Work out the finished part from the listing and answer in its coordinate system (mm). Round coordinates to 2 decimals unless told otherwise and drop trailing zeros. Loops run counter-clockwise (first coordinate to the right, second up) from the corner with the lowest first, then second, coordinate; pieces in that order, holes last. Notation, with made-up numbers: (23.5, -24) -> (72.5, -24) arc R23 ccw to (72.5, -1) -> close; hole circle Ø10 at (4.25, 24). An arc over 180 degrees is marked (long way). Use CSV: the item, a comma, the result in double quotes. Start each with the question number.
Autodesk Fusion 360 part; units mm, degrees
sketch "Esquisse1" plane through (0, 0, 0) normal (0, 0, 1) x (1, 0, 0)
  line L0 (-15, 10) -> (15, 10)
  line L1 (15, 10) -> (15, 0)
  line L2 (15, 0) -> (-15, 0)
  line L3 (-15, 0) -> (-15, 10)
  line L4 (0, 1.75) -> (0, 22.5)
  dimension "d1" = 30
  dimension "d2" = 10
extrude "Extrusion1" add sketch "Esquisse1" along normal blind 46
sketch "Esquisse2" plane through (0, 0, 0) normal (0, 0, -1) x (1, 0, 0)
  line L0 (15, 0) -> (-15, 0)
  line L1 (-15, 0) -> (-15, -10)
  line L2 (-15, -10) -> (15, -10)
  line L3 (15, -10) -> (15, 0)
  point P0 (-11, -5)
  dimension "d5" = 11
  dimension "d6" = 5
hole "Perçage1" at (-11, 5, 0) direction (0, 0, 1) diameter 2.5 depth 57 tip angle 118
mirror "Symétrie miroir1" about plane through (0, 0, 0) normal (1, 0, 0) of "Perçage1"
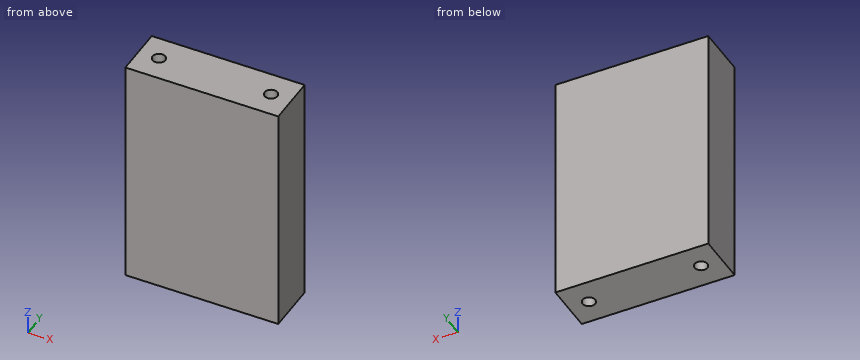
Q1. Straight lines are drawn through the part: line 1 (X direction, y = 5, z = 21.5); line 2 (Y direction, x = -11, z = 26.5); line 3 (X direction, y = 5.75, z = 7). For each, find the intervals that lie inside material, in ascending order. Write a range as from..to.
Q2. Section B-B, the plane y = 5 is taken. Write down the section's boundary in (x, z).
Q3. Section A-A, the plane x = -11 is taken. Write down the section's boundary in (y, z).
Q4. Section C-C, the plane z = 17.5 is taken. Write down the section's boundary in (x, y).
Report:
1,line 1,"x = -15..-12.25, -9.75..9.75, 12.25..15"
1,line 2,"y = 0..3.75, 6.25..10"
1,line 3,"x = -15..-12, -10..10, 12..15"
2,outline,"(-15, 0) -> (-12.25, 0) -> (-12.25, 46) -> (-15, 46) -> close; (-9.75, 0) -> (9.75, 0) -> (9.75, 46) -> (-9.75, 46) -> close; (12.25, 0) -> (15, 0) -> (15, 46) -> (12.25, 46) -> close"
3,outline,"(0, 0) -> (3.75, 0) -> (3.75, 46) -> (0, 46) -> close; (6.25, 0) -> (10, 0) -> (10, 46) -> (6.25, 46) -> close"
4,outline,"(-15, 0) -> (15, 0) -> (15, 10) -> (-15, 10) -> close; hole circle Ø2.5 at (-11, 5); hole circle Ø2.5 at (11, 5)"
